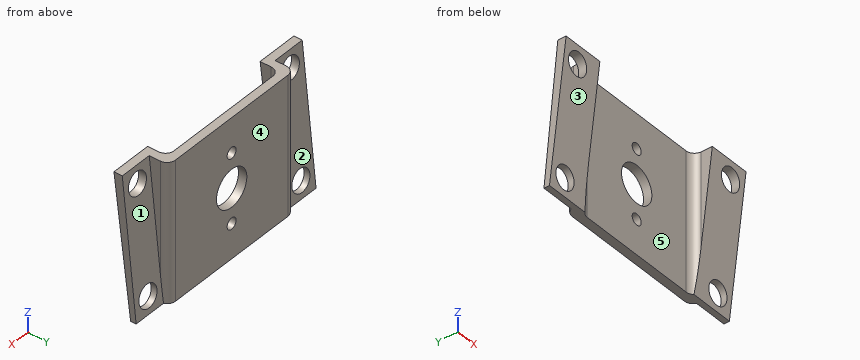
from build123d import *

# Parameters (mm, degrees)
F0_W     = 50
F0_H     = 50
F0_R     = 2
F0_R_2   = 6.75
F1_DEPTH = 3
F3_START = 25
F3_DEPTH = 3
F5_START = -25
F5_DEPTH = 3
F7_START = 25
F7_DEPTH = 15
F8_START = -25
F8_DEPTH = 15
F10_D    = 8
F11_R    = 3


with BuildPart() as f1:
    # F0 (on Front) → F1 (new body)
    with BuildSketch(Plane.XZ):
        Rectangle(F0_W, F0_H)
        with Locations((0, -12.5)):
            Circle(F0_R, mode=Mode.SUBTRACT)
        Circle(F0_R_2, mode=Mode.SUBTRACT)
        with Locations((0, 12.5)):
            Circle(F0_R, mode=Mode.SUBTRACT)
    extrude(amount=F1_DEPTH)

    # F2 (on Right) → F3 (join)
    with BuildSketch(Plane.YZ.offset(F3_START)):
        Polygon((0, 25), (-2, 25), (-7, 25), (-2, -25), (0, -25), align=None)
    extrude(amount=F3_DEPTH)

    # F4 (on Right) → F5 (join)
    with BuildSketch(Plane.YZ.offset(F5_START)):
        Polygon((0, -25), (0, 25), (-2, 25), (-7, 25), (-2, -25), align=None)
    extrude(amount=-F5_DEPTH)

    # F6 (on Right) → F7 (join)
    with BuildSketch(Plane.YZ.offset(F7_START)):
        Polygon((-2, -25), (-7, 25), (-10, 25), (-4, -25), align=None)
    extrude(amount=F7_DEPTH)

    # F6 (on Right) → F8 (join)
    with BuildSketch(Plane.YZ.offset(F8_START)):
        Polygon((-2, -25), (-7, 25), (-10, 25), (-4, -25), align=None)
    extrude(amount=-F8_DEPTH)

    # F10 (through all)
    with Locations(Plane(origin=(0, 0, 0), x_dir=(1, 0, 0), z_dir=(0, 1, 0))):
        with Locations((-34, -19), (-34, 19), (34, 19), (34, -19)):
            Hole(F10_D / 2)

    # F11
    f11_edges = [f1.edges().sort_by_distance(p)[0] for p in [
        (-28, 0, 0),
        (28, 0, 0),
        (25, -3, 0),
        (-25, -3, 0),
    ]]
    fillet(f11_edges, radius=F11_R)


solid = f1.part
Work out the finished part from the listing and answer in its coordinate system (mm). Face numbers are marked on the shaded views. A direction names the side the tool comes from. Round coordinates to 2 decimals unless told otherwise and drop trailing zeros. Write each loop counter-clockwise with the first axis right and the second up, starting at its lowest first coordinate (ties: lowest second). Pieces come first, ordered by that corner, then holes.
1) A cutting plane is placed at C-C (z = 19). Give the vertices of the cut face in (x, y), plus the area to 3 significant figures.
2) Given pin 1 Ø7 at (x, z) = (34, -19) entering from -Y; pin 2 Ø6 at (x, z) = (-4, -1.5) entering from -Y; pin 3 Ø13 at (x, z) = (34, 19) entering from +Y; pin 4 Ø6 at (y, z) = (-1.5, 4) entering from +X, each flat-ended and moving along its own axis, determine where each tip first touches the part or whether it passes through.
3) A tool of negligible diameter and unlimited length cuts with its end or side. For the marked faces 1, 2 and 3, from which of +Z, -Z, +X, -X, +Y, -Y can it reach the whole face along a straight path? Write none if from no direction.
4) A cutting plane is placed at D-D (x = 34). Give the vertices of the cut face in (y, z), plus the area to 3 significant figures.
5) The mould has two halves that part along X. Classify the marked faces 4 and 5: pulls with the +X half, pulls with the -X half, needs draft (parallel to the pull), parting line crosses it, or undercut.
6) A cutting plane is placed at B-B (x = 0). Give the vertices of the cut face in (y, z).
7) A cutting plane is placed at A-A (z = 0). Give the vertices of the cut face in (x, y), plus the area to 4 significant figures.
8) Straight lines are drawn through the part: line 1 (Z direction, x = 0, y = -1.5); line 2 (X direction, y = -8, z = 19); line 3 (X direction, y = -2.95, z = -19). For each, find the intervals that lie inside material, in ascending order.
Completed:
1. outline: (-40, -9.28) - (-38, -9.28) - (-38, -6.4) - (-40, -6.4) - close; (-30, -9.28) - (-25, -9.28) - (-25, -6) arc R3 cw to (-22, -3) - (22, -3) arc R3 cw to (25, -6) - (25, -9.28) - (30, -9.28) - (30, -6.4) - (28, -6.4) - (28, -3) arc R3 ccw to (25, 0) - (-25, 0) arc R3 ccw to (-28, -3) - (-28, -6.4) - (-30, -6.4) - close; (38, -9.28) - (40, -9.28) - (40, -6.4) - (38, -6.4) - close
1. area: 229 mm2
2. pin 1: passes through
2. pin 2: stops at y = -3
2. pin 3: stops at y = -1.34
2. pin 4: stops at x = 28
3. face 1: +Z, +X, +Y
3. face 2: +Z, -X, +Y
3. face 3: -Z, +X, -X, -Y
4. outline: (-10, 25) - (-9.76, 23) - (-6.8, 23) - (-7, 25) - close; (-8.8, 15) - (-5.2, -15) - (-3, -15) - (-6, 15) - close; (-4.24, -23) - (-4, -25) - (-2, -25) - (-2.2, -23) - close
4. area: 85.0 mm2
5. face 4: needs draft
5. face 5: undercut
6. outline: (-3, -25) - (0, -25) - (0, -14.5) - (-3, -14.5) - close; (-3, -10.5) - (0, -10.5) - (0, -6.75) - (-3, -6.75) - close; (-3, 6.75) - (0, 6.75) - (0, 10.5) - (-3, 10.5) - close; (-3, 14.5) - (0, 14.5) - (0, 25) - (-3, 25) - close
7. outline: (-40, -7) - (-25, -7) - (-25, -6) arc R3 cw to (-22, -3) - (-6.75, -3) - (-6.75, 0) - (-25, 0) arc R3 ccw to (-28, -3) - (-28, -4.5) - (-40, -4.5) - close; (6.75, -3) - (22, -3) arc R3 cw to (25, -6) - (25, -7) - (40, -7) - (40, -4.5) - (28, -4.5) - (28, -3) arc R3 ccw to (25, 0) - (6.75, 0) - close
7. area: 211.5 mm2
8. line 1: z = -25 to -14.5, -10.5 to -6.75, 6.75 to 10.5, 14.5 to 25
8. line 2: x = -40 to -38, -30 to -25, 25 to 30, 38 to 40
8. line 3: x = -40 to -38, -30 to 30, 38 to 40
